Check sheet for the drawn part. Datum: minimum x, y, z corner. Units: mm. Give positions to 0.01 mm unless a question says otherwise; leave off trailing zeros. Order: outer loops, then holes, each group sorted by start corner. A loop starts at its lowest first (then second) coordinate and runs counter-clockwise, first axis right, second up.
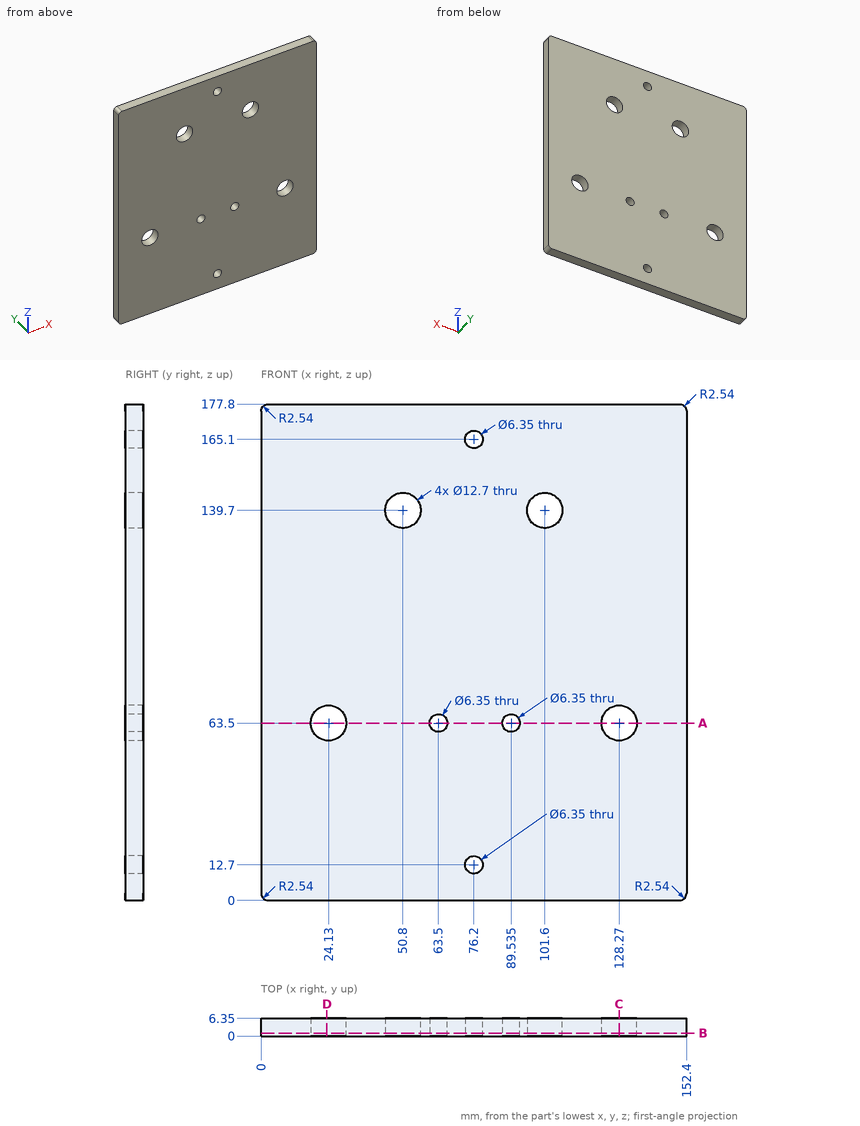
Item 1: Gauge pin test, flat end, axial feed: pin 1 (10 mm diameter, centred on x = 128.27, z = 63.5, fed in from -Y). Record the tip position at first contact, or that the pin passes through.
Reported:
pin 1: passes through
Item 2: Sectioned sample at B-B (y = 1). Give the number of separate pieces and of enclosed holes in the cut face, and give its area (3 significant figures).
Reported:
separate pieces: 1
enclosed holes: 8
area: 26,500 mm2
Item 3: Sectioned sample at A-A (z = 63.5). Enter the section's corners in (x, y) (3 decimals).
Reported:
outline: (0, 0) - (17.78, 0) - (17.78, 6.35) - (0, 6.35) - close; (30.48, 0) - (60.325, 0) - (60.325, 6.35) - (30.48, 6.35) - close; (66.675, 0) - (86.36, 0) - (86.36, 6.35) - (66.675, 6.35) - close; (92.71, 0) - (121.92, 0) - (121.92, 6.35) - (92.71, 6.35) - close; (134.62, 0) - (152.4, 0) - (152.4, 6.35) - (134.62, 6.35) - close
Item 4: Scan lines: L1, parallel to Z at x = 50.8, y = 2.5; L2, parallel to X at y = 2.25, z = 139.5; L3, parallel to Z at x = 63.5, y = 2.5 (3 decimals). Record each from-to range of solid material in increasing order.
Reported:
L1: z = 0 to 133.35, 146.05 to 177.8
L2: x = 0 to 44.45, 57.15 to 95.25, 107.95 to 152.4
L3: z = 0 to 60.325, 66.675 to 177.8
Item 5: Sectioned sample at C-C (x = 128.27). Enter the section's corners in (y, z), and give its area (3 significant figures).
Reported:
outline: (0, 0) - (6.35, 0) - (6.35, 57.15) - (0, 57.15) - close; (0, 69.85) - (6.35, 69.85) - (6.35, 177.8) - (0, 177.8) - close
area: 1,050 mm2
Item 6: Sectioned sample at D-D (x = 23.5). Enter the section's corners in (y, z), and give its area (3 significant figures).
Reported:
outline: (0, 0) - (6.35, 0) - (6.35, 57.18) - (0, 57.18) - close; (0, 69.82) - (6.35, 69.82) - (6.35, 177.8) - (0, 177.8) - close
area: 1,050 mm2
